Could you check a few things on this model? Use its own coordinates, in mm. A direction names the side the tool comes from. Coordinates: 2 decimals unless noted, no trailing zeros. Order: outer loops, then holes, each group sorted by start corner. A loop starts at its lowest first (then second) coordinate and runs counter-clockwise, first axis right, second up. Notation, with made-up numbers: (65.25, -13.75) - (108.25, -13.75) arc R29 ccw to (108.25, 25.25) - close; hole circle Ø7 at (66.25, 18.5). An arc over 180 degrees is marked (long way). Answer as CSV lines item,"result". Start each with the question number.
1. For pin 1 (3.5 mm diameter, centred on x = 15.27, y = -23.97, fed in from -Z); pin 2 (6 mm diameter, centred on x = 6, y = -4.5, fed in from -Z); pin 3 (2 mm diameter, centred on x = 15, z = -6, fed in from -Y), each with a flat end and sliding along its axis, tell me the tip position at first contact or that it passes through.
2. I want a section at C-C, the plane y = 24. List the corners of the cut face in (x, z) for me.
3. I want a section at D-D, the plane x = 4.5. List the corners of the cut face in (y, z) for me.
4. Thinking about a two-plate mould opening in Y: for faces 4 (the face through (10, -24, -31.5)), 5 (the face through (4.77, -21.92, 0.04)), 6 (the face through (10, 27.5, -15)), which applies, released by +Y, released by -Y, zero draft, split by the parting line, or undercut?
5. I want a section at B-B, the plane x = 15.25. List the corners of the cut face in (y, z) for me.
6. I need wall thicknesses on probe 1 along Y at (x, z) = (5.25, -28.05); probe 2 along Y at (x, z) = (15.25, 0.1); probe 3 along Y at (x, z) = (17.75, -11). Which ranges of each line are inside material? Lowest first, please.
7. For faces 1 (the face through (4.12, 25.77, -29.04)), 2 (the face through (10, 20.5, -17)), 3 (the face through (16.38, 22.23, 0.04)), which set-ups out of +Z, -Z, +X, -X, +Y, -Y let a thin tool reach every point of the face, with its end or its side?
8. I want a section at A-A, the plane z = -16. List the corners of the cut face in (x, y) for me.
from build123d import *

# Parameters (mm, degrees)
BOSS_EXTRUDE1_DEPTH = 20.5
SKETCH3_W           = 13.820879987
SKETCH3_H           = 19.579579981
CUT_EXTRUDE1_DEPTH  = 7
SKETCH4_R           = 2.1
CUT_EXTRUDE2_DEPTH  = 5


with BuildPart() as part:
    # Sketch1 → Boss-Extrude1 (new body)
    with BuildSketch(Plane(origin=(0, 0, 0), x_dir=(0, 0, -1), z_dir=(1, 0, 0))):
        Polygon((-2.5, 27.5), (2.5, 27.5), (31.5, 27.5), (31.5, 20.5), (2.5, 20.5), (2.5, -20.5), (31.5, -20.5), (31.5, -27.5), (2.5, -27.5), (-2.5, -27.5), align=None)
    extrude(amount=BOSS_EXTRUDE1_DEPTH)

    # Sketch3 → Cut-Extrude1 (cut)
    with BuildSketch(Plane.XZ.offset(27.5)):
        with Locations((10.385498824, -12.910906187)):
            Rectangle(SKETCH3_W, SKETCH3_H)
    extrude(amount=-CUT_EXTRUDE1_DEPTH, mode=Mode.SUBTRACT)

    # Sketch4 → Cut-Extrude2 (cut)
    with BuildSketch(Plane(origin=(0, 0, -31.5), x_dir=(-1, 0, 0), z_dir=(0, 0, -1))):
        with Locations((-15.271378587, -23.970399076)):
            Circle(SKETCH4_R)
        with Locations(Location((-5.228621413, -23.970399076, 0), (0, 0, 180))):
            Circle(SKETCH4_R)
        with Locations((-5.25, 24)):
            Circle(SKETCH4_R)
        with Locations(Location((-15.25, 24, 0), (0, 0, 180))):
            Circle(SKETCH4_R)
    cut_extrude2 = extrude(amount=-CUT_EXTRUDE2_DEPTH, mode=Mode.SUBTRACT)

    # Mirror1: Cut-Extrude2 across plane
    add(cut_extrude2.mirror(Plane.XY.offset(-14.5)), mode=Mode.SUBTRACT)


solid = part.part
Solved:
1,pin 1,"stops at z = -26.5"
1,pin 2,"stops at z = -2.5"
1,pin 3,"stops at y = 20.5"
2,outline,"(0, -31.5) - (3.15, -31.5) - (3.15, -26.5) - (7.35, -26.5) - (7.35, -31.5) - (13.15, -31.5) - (13.15, -26.5) - (17.35, -26.5) - (17.35, -31.5) - (20.5, -31.5) - (20.5, 2.5) - (17.35, 2.5) - (17.35, -2.5) - (13.15, -2.5) - (13.15, 2.5) - (7.35, 2.5) - (7.35, -2.5) - (3.15, -2.5) - (3.15, 2.5) - (0, 2.5) - close"
3,outline,"(-27.5, -31.5) - (-25.94, -31.5) - (-25.94, -26.5) - (-22, -26.5) - (-22, -31.5) - (-20.5, -31.5) - (-20.5, -22.7) - (-27.5, -22.7) - close; (-27.5, -3.12) - (-20.5, -3.12) - (-20.5, -2.5) - (20.5, -2.5) - (20.5, -31.5) - (22.04, -31.5) - (22.04, -26.5) - (25.96, -26.5) - (25.96, -31.5) - (27.5, -31.5) - (27.5, 2.5) - (25.96, 2.5) - (25.96, -2.5) - (22.04, -2.5) - (22.04, 2.5) - (-22, 2.5) - (-22, -2.5) - (-25.94, -2.5) - (-25.94, 2.5) - (-27.5, 2.5) - close"
4,face 4,"zero draft"
4,face 5,"undercut"
4,face 6,"released by +Y"
5,outline,"(-27.5, -31.5) - (-26.07, -31.5) - (-26.07, -26.5) - (-21.87, -26.5) - (-21.87, -31.5) - (-20.5, -31.5) - (-20.5, -22.7) - (-27.5, -22.7) - close; (-27.5, -3.12) - (-20.5, -3.12) - (-20.5, -2.5) - (20.5, -2.5) - (20.5, -31.5) - (21.9, -31.5) - (21.9, -26.5) - (26.1, -26.5) - (26.1, -31.5) - (27.5, -31.5) - (27.5, 2.5) - (26.1, 2.5) - (26.1, -2.5) - (21.9, -2.5) - (21.9, 2.5) - (-21.87, 2.5) - (-21.87, -2.5) - (-26.07, -2.5) - (-26.07, 2.5) - (-27.5, 2.5) - close"
6,probe 1,"y = -27.5 to -26.07, -21.87 to -20.5, 20.5 to 21.9, 26.1 to 27.5"
6,probe 2,"y = -27.5 to -26.07, -21.87 to 21.9, 26.1 to 27.5"
6,probe 3,"y = -27.5 to -20.5, 20.5 to 27.5"
7,face 1,"-Z"
7,face 2,"-Z, +X, -X"
7,face 3,"+Z"
8,outline,"(0, -27.5) - (3.48, -27.5) - (3.48, -20.5) - (0, -20.5) - close; (0, 20.5) - (20.5, 20.5) - (20.5, 27.5) - (0, 27.5) - close; (17.3, -27.5) - (20.5, -27.5) - (20.5, -20.5) - (17.3, -20.5) - close"
